```python
from build123d import *

# Parameters (mm, degrees)
CROQUIS1_W              = 55.55
CROQUIS1_H              = 20.1
SALIENTE_EXTRUIR1_DEPTH = 2
CROQUIS2_R              = 2
CORTAR_EXTRUIR1_DEPTH   = 30.604951022
CROQUIS3_W              = 2
CROQUIS3_H              = 20.1
SALIENTE_EXTRUIR2_DEPTH = 35
CORTAR_EXTRUIR2_REACH   = 68.421
CROQUIS4_R              = 4
CROQUIS4_R_2            = 1.45
REDONDEO4_R             = 10


with BuildPart() as part:
    # Croquis1 → Saliente-Extruir1 (new body)
    with BuildSketch(Plane.XY):
        Rectangle(CROQUIS1_W, CROQUIS1_H)
    extrude(amount=SALIENTE_EXTRUIR1_DEPTH)

    # Croquis2 → Cortar-Extruir1 (cut, through all)
    with BuildSketch(Plane.XY.offset(2)):
        Circle(CROQUIS2_R)
        with Locations((5, 5)):
            Circle(CROQUIS2_R)
        with Locations((5, -5)):
            Circle(CROQUIS2_R)
        with Locations(Location((-5, -5, 0), (0, 0, 180))):
            Circle(CROQUIS2_R)
        with Locations(Location((-5, 5, 0), (0, 0, 180))):
            Circle(CROQUIS2_R)
        with Locations((15, 5)):
            Circle(CROQUIS2_R)
        with Locations((15, -5)):
            Circle(CROQUIS2_R)
        with Locations(Location((-15, 5, 0), (0, 0, 180))):
            Circle(CROQUIS2_R)
        with Locations(Location((-15, -5, 0), (0, 0, 180))):
            Circle(CROQUIS2_R)
    extrude(amount=-CORTAR_EXTRUIR1_DEPTH, mode=Mode.SUBTRACT)

    # Croquis3 → Saliente-Extruir2 (add)
    with BuildSketch(Plane.XY):
        with Locations((-26.775, 0)):
            Rectangle(CROQUIS3_W, CROQUIS3_H)
        with Locations((26.775, 0)):
            Rectangle(CROQUIS3_W, CROQUIS3_H)
    extrude(amount=SALIENTE_EXTRUIR2_DEPTH)

    # Cortar-Extruir2: up to this face of the body (flat: up to its plane)
    cortar_extruir2_end = Plane(part.part.faces().sort_by_distance((-27.775, 0, 17.5))[0])
    # Croquis4 → Cortar-Extruir2 (cut, up to the picked face)
    with BuildSketch(Plane(origin=(27.775, 0, 0), x_dir=(0, 0, -1), z_dir=(1, 0, 0)), mode=Mode.PRIVATE) as cortar_extruir2_sk1:
        with Locations((-25, 0)):
            Circle(CROQUIS4_R)
    cortar_extruir2_tool1 = split(extrude(cortar_extruir2_sk1.sketch, amount=-CORTAR_EXTRUIR2_REACH, mode=Mode.PRIVATE), bisect_by=cortar_extruir2_end, keep=Keep.BOTH, mode=Mode.PRIVATE)
    # Croquis4 → Cortar-Extruir2 (cut, up to the picked face)
    with BuildSketch(Plane(origin=(27.775, 0, 0), x_dir=(0, 0, -1), z_dir=(1, 0, 0)), mode=Mode.PRIVATE) as cortar_extruir2_sk2:
        with Locations((-32.05, 0)):
            Circle(CROQUIS4_R_2)
    cortar_extruir2_tool2 = split(extrude(cortar_extruir2_sk2.sketch, amount=-CORTAR_EXTRUIR2_REACH, mode=Mode.PRIVATE), bisect_by=cortar_extruir2_end, keep=Keep.BOTH, mode=Mode.PRIVATE)
    # Croquis4 → Cortar-Extruir2 (cut, up to the picked face)
    with BuildSketch(Plane(origin=(27.775, 0, 0), x_dir=(0, 0, -1), z_dir=(1, 0, 0)), mode=Mode.PRIVATE) as cortar_extruir2_sk3:
        with Locations(Location((-17.95, 0, 0), (0, 0, 90))):
            Circle(CROQUIS4_R_2)
    cortar_extruir2_tool3 = split(extrude(cortar_extruir2_sk3.sketch, amount=-CORTAR_EXTRUIR2_REACH, mode=Mode.PRIVATE), bisect_by=cortar_extruir2_end, keep=Keep.BOTH, mode=Mode.PRIVATE)
    # Croquis4 → Cortar-Extruir2 (cut, up to the picked face)
    with BuildSketch(Plane(origin=(27.775, 0, 0), x_dir=(0, 0, -1), z_dir=(1, 0, 0)), mode=Mode.PRIVATE) as cortar_extruir2_sk4:
        with Locations(Location((-20.014897193, -4.985102807, 0), (0, 0, 90))):
            Circle(CROQUIS4_R_2)
    cortar_extruir2_tool4 = split(extrude(cortar_extruir2_sk4.sketch, amount=-CORTAR_EXTRUIR2_REACH, mode=Mode.PRIVATE), bisect_by=cortar_extruir2_end, keep=Keep.BOTH, mode=Mode.PRIVATE)
    # Croquis4 → Cortar-Extruir2 (cut, up to the picked face)
    with BuildSketch(Plane(origin=(27.775, 0, 0), x_dir=(0, 0, -1), z_dir=(1, 0, 0)), mode=Mode.PRIVATE) as cortar_extruir2_sk5:
        with Locations(Location((-25, -7.05, 0), (0, 0, 90))):
            Circle(CROQUIS4_R_2)
    cortar_extruir2_tool5 = split(extrude(cortar_extruir2_sk5.sketch, amount=-CORTAR_EXTRUIR2_REACH, mode=Mode.PRIVATE), bisect_by=cortar_extruir2_end, keep=Keep.BOTH, mode=Mode.PRIVATE)
    # Croquis4 → Cortar-Extruir2 (cut, up to the picked face)
    with BuildSketch(Plane(origin=(27.775, 0, 0), x_dir=(0, 0, -1), z_dir=(1, 0, 0)), mode=Mode.PRIVATE) as cortar_extruir2_sk6:
        with Locations((-25, 7.05)):
            Circle(CROQUIS4_R_2)
    cortar_extruir2_tool6 = split(extrude(cortar_extruir2_sk6.sketch, amount=-CORTAR_EXTRUIR2_REACH, mode=Mode.PRIVATE), bisect_by=cortar_extruir2_end, keep=Keep.BOTH, mode=Mode.PRIVATE)
    # Croquis4 → Cortar-Extruir2 (cut, up to the picked face)
    with BuildSketch(Plane(origin=(27.775, 0, 0), x_dir=(0, 0, -1), z_dir=(1, 0, 0)), mode=Mode.PRIVATE) as cortar_extruir2_sk7:
        with Locations((-20.014897193, 4.985102807)):
            Circle(CROQUIS4_R_2)
    cortar_extruir2_tool7 = split(extrude(cortar_extruir2_sk7.sketch, amount=-CORTAR_EXTRUIR2_REACH, mode=Mode.PRIVATE), bisect_by=cortar_extruir2_end, keep=Keep.BOTH, mode=Mode.PRIVATE)
    add(cortar_extruir2_tool1.solids().sort_by(Axis((27.775, 0, 25), (-1, 0, 0)))[0], mode=Mode.SUBTRACT)
    add(cortar_extruir2_tool2.solids().sort_by(Axis((27.775, 0, 32.05), (-1, 0, 0)))[0], mode=Mode.SUBTRACT)
    add(cortar_extruir2_tool3.solids().sort_by(Axis((27.775, 0, 17.95), (-1, 0, 0)))[0], mode=Mode.SUBTRACT)
    add(cortar_extruir2_tool4.solids().sort_by(Axis((27.775, -4.985103, 20.014897), (-1, 0, 0)))[0], mode=Mode.SUBTRACT)
    add(cortar_extruir2_tool5.solids().sort_by(Axis((27.775, -7.05, 25), (-1, 0, 0)))[0], mode=Mode.SUBTRACT)
    add(cortar_extruir2_tool6.solids().sort_by(Axis((27.775, 7.05, 25), (-1, 0, 0)))[0], mode=Mode.SUBTRACT)
    add(cortar_extruir2_tool7.solids().sort_by(Axis((27.775, 4.985103, 20.014897), (-1, 0, 0)))[0], mode=Mode.SUBTRACT)

    # Redondeo4
    redondeo4_edges = [part.edges().sort_by_distance(p)[0] for p in [
        (-26.775, -10.05, 35),
        (-26.775, 10.05, 35),
        (26.775, 10.05, 35),
        (26.775, -10.05, 35),
    ]]
    fillet(redondeo4_edges, radius=REDONDEO4_R)


solid = part.part
```
CAD build for the part. Positions are in the model's coordinates, mm. A direction names the side the tool comes from. Round coordinates to 2 decimals unless told otherwise and drop trailing zeros. Order: outer loops, then holes, each group sorted by start corner. A loop starts at its lowest first (then second) coordinate and runs counter-clockwise, first axis right, second up.
Q1. Wall check: L1, parallel to X at y = -3.25, z = 14 (3 decimals); L2, parallel to Z at x = -25, y = 1.5. Give the ranges that are in metal, low to high.
Q2. Slice it at B-B (z = 4). Write the cut outline in (x, y) (3 decimals), and give its area (3 significant figures).
Q3. Slice it at C-C (y = -5). State how many separate pieces and enclosed holes the cut face has, and give its area (3 significant figures).
Q4. Slice it at D-D (x = -14). Write the cut outline in (y, z).
Q5. Which spindle directions (+Z, -Z, +X, -X, +Y, -Y) get a long thin tool onto all of the face, cutting with end or side? Do faces 1 (the cylindrical face through (-13.4, 6.2, 1)), 2 (the flat face through (-0.4, 2.4, 2)). Say none if no direction does.
Q6. Two-plate mould, pull along X, no slides. Class faces 3 (the flat face through (-2, -10.05, 1)), 4 (the cylindrical face through (3.4, -6.2, 1)): pulls with the +X half, pulls with the -X half, needs draft (parallel to the pull), parting line crosses it, or undercut.
Q7. Drop flat-ended pins along their axis: pin 1 (7 mm diameter, centred on y = 0, z = 25, fed in from -X); pin 2 (1 mm diameter, centred on x = -14.5, y = 3.5, fed in from +Z). Give the stop position or say it passes through.
Q8. Slice it at A-A (x = 0). Write the cut outline in (y, z), and give its area (3 significant figures).
Results below:
1. L1: x = -27.775 to -25.775, 25.775 to 27.775
1. L2: z = 0 to 2
2. outline: (-27.775, -10.05) - (-25.775, -10.05) - (-25.775, 10.05) - (-27.775, 10.05) - close; (25.775, -10.05) - (27.775, -10.05) - (27.775, 10.05) - (25.775, 10.05) - close
2. area: 80.4 mm2
3. separate pieces: 7
3. enclosed holes: 0
3. area: 194 mm2
4. outline: (-10.05, 0) - (-6.73, 0) - (-6.73, 2) - (-10.05, 2) - close; (-3.27, 0) - (3.27, 0) - (3.27, 2) - (-3.27, 2) - close; (6.73, 0) - (10.05, 0) - (10.05, 2) - (6.73, 2) - close
5. face 1: +Z, -Z
5. face 2: +Z, +Y, -Y
6. face 3: needs draft
6. face 4: undercut
7. pin 1: passes through
7. pin 2: stops at z = 2
8. outline: (-10.05, 0) - (-2, 0) - (-2, 2) - (-10.05, 2) - close; (2, 0) - (10.05, 0) - (10.05, 2) - (2, 2) - close
8. area: 32.2 mm2
